Geometry: final body of the model. Coordinates: model frame, mm. A direction names the side the tool comes from. Round coordinates to 2 decimals unless told otherwise and drop trailing zeros. Loops run counter-clockwise (first coordinate to the right, second up) from the corner with the lowest first, then second, coordinate; pieces in that order, holes last. Notation, with made-up numbers: (-9, 79) - (22, 79) arc R21 cw to (22, 92) - close; hole circle Ø4 at (-40, -23.75). An arc over 180 degrees is marked (long way). Return JSON: item names as keys, results as strings. Group by question number.
1. Set-up query: faces 1 (the face through (-1, 0, 5)), 2 (the face through (14.53, 14.55, 2.54)), 3 (the face through (37, 27.5, 3)). Return all of +Z, -Z, +X, -X, +Y, -Y with unobstructed straight access to the full face (end or side cutting, diameter ignored); none if empty.
2. Material intervals for probe 1 along X at (y, z) = (12, 13); probe 2 along Y at (x, z) = (-1.5, 7); probe 3 along X at (y, z) = (18, 4.5), sorted ascending.
3. Section B-B on x = -50. Return loops of the section in (y, z), and give its area (3 significant figures).
4. Section D-D on x = 7.5. Return loops of the section in (y, z).
5. Section A-A on z = 18.5. Return loops of the section in (x, y), and give its area (3 significant figures).
6. Draft query along X for faces 4 (the face through (21.86, 9.83, 2.54)), 5 (the face through (-20, 29, 4)), 6 (the face through (0, 30.5, 4)). Return one class per face: +X half, -X half, draft (parallel to the pull), parting line (faces both ways), or undercut.
7. First-contact query: pin 1 Ø6 at (x, y) = (33.5, -0.5) entering from +Z; pin 2 Ø1.5 at (y, z) = (29, 2) entering from +X; pin 3 Ø3.5 at (y, z) = (29, 2.5) entering from -X. Flat tips, straight axial feed; report the tip coordinate or a pass-through.
from build123d import *

# Parameters (mm, degrees)
SKETCH1_W             = 82
SKETCH1_H             = 55
BOSS_EXTRUDE1_DEPTH   = 5
SKETCH1_W_2           = 12
BOSS_EXTRUDE1_2_DEPTH = 5
BOSS_EXTRUDE1_3_DEPTH = 5
SKETCH1_3_W           = 2
SKETCH1_3_H           = 55
BOSS_EXTRUDE2_DEPTH   = 7
FILLET1_R             = 1
SKETCH2_W             = 5
SKETCH2_H             = 45
BOSS_EXTRUDE3_DEPTH   = 16
SKETCH3_W             = 17
SKETCH3_H             = 45
BOSS_EXTRUDE4_DEPTH   = 5
SKETCH4_W             = 40
SKETCH4_H             = 3
BOSS_EXTRUDE5_DEPTH   = 8
CUT_EXTRUDE1_DEPTH    = 8


with BuildPart() as part:
    # Sketch1 → Boss-Extrude1 (new body)
    with BuildSketch(Plane.XY):
        Rectangle(SKETCH1_W, SKETCH1_H)
    extrude(amount=BOSS_EXTRUDE1_DEPTH)



with BuildPart() as body_2:
    # Sketch1 → Boss-Extrude1 2 (new body)
    with BuildSketch(Plane.XY):
        with Locations((-49, 0)):
            Rectangle(SKETCH1_W_2, SKETCH1_H)
    extrude(amount=BOSS_EXTRUDE1_2_DEPTH)


with BuildPart() as body_3:
    # Sketch1 → Boss-Extrude1 3 (new body)
    with BuildSketch(Plane.XY):
        with Locations((49, 0)):
            Rectangle(SKETCH1_W_2, SKETCH1_H)
    extrude(amount=BOSS_EXTRUDE1_3_DEPTH)


with BuildPart() as part_1:
    add(part.part)

    add(body_2.part)  # Boss-Extrude2 merges body 2

    add(body_3.part)  # Boss-Extrude2 merges body 3
    # Sketch1<3> → Boss-Extrude2 (add)
    with BuildSketch(Plane.XY):
        with Locations((42, 0)):
            Rectangle(SKETCH1_3_W, SKETCH1_3_H)
        with Locations((-42, 0)):
            Rectangle(SKETCH1_3_W, SKETCH1_3_H)
    extrude(amount=BOSS_EXTRUDE2_DEPTH)

    # Fillet1
    fillet1_edges = [part_1.edges().sort_by_distance(p)[0] for p in [
        (-43, 0, 7),
        (-41, 0, 7),
        (41, 0, 7),
        (43, 0, 7),
    ]]
    fillet(fillet1_edges, radius=FILLET1_R - 0.0001)  # a hair under: the kernel refuses the full size

    # Sketch2 → Boss-Extrude3 (add)
    with BuildSketch(Plane.XY):
        with Locations((-57.5, 0)):
            Rectangle(SKETCH2_W, SKETCH2_H)
        with Locations((57.5, 0)):
            Rectangle(SKETCH2_W, SKETCH2_H)
    extrude(amount=BOSS_EXTRUDE3_DEPTH)

    # Sketch3 → Boss-Extrude4 (add)
    with BuildSketch(Plane.XY.offset(16)):
        with Locations((51.5, 0)):
            Rectangle(SKETCH3_W, SKETCH3_H)
        with Locations((-51.5, 0)):
            Rectangle(SKETCH3_W, SKETCH3_H)
    extrude(amount=BOSS_EXTRUDE4_DEPTH)

    # Sketch4 → Boss-Extrude5 (add)
    with BuildSketch(Plane.XY):
        with Locations((0, -29)):
            Rectangle(SKETCH4_W, SKETCH4_H)
        with Locations((0, 29)):
            Rectangle(SKETCH4_W, SKETCH4_H)
    extrude(amount=BOSS_EXTRUDE5_DEPTH)

    # Sketch5 → Cut-Extrude1 (cut)
    with BuildSketch(Plane.XY.offset(5)):
        Polygon((32.5, -2.5), (11.171238341, -2.5), (32.5, -16.386089579), align=None)
        Polygon((26.151212641, -21.798780488), (4, -7.377234224), (4, -21.798780488), align=None)
        Polygon((-4, -7.494684737), (-25.350036879, -21.798780488), (-4, -21.798780488), align=None)
        Polygon((-10.917888224, -2.5), (-32.5, -2.5), (-32.5, -16.959581269), align=None)
        Polygon((-11.171238341, 2.5), (-32.5, 16.386089579), (-32.5, 2.5), align=None)
        Polygon((-4, 21.798780488), (-26.151212641, 21.798780488), (-4, 7.377234224), align=None)
        Polygon((25.350035913, 21.798780488), (4, 21.798780488), (4, 7.494685385), align=None)
        Polygon((32.5, 2.5), (32.5, 16.959581917), (10.917887257, 2.5), align=None)
    extrude(amount=-CUT_EXTRUDE1_DEPTH, mode=Mode.SUBTRACT)


solid = part_1.part
Taken from the geometry:
{
 "1": {"face 1": "+Z", "face 2": "+Z, -Z", "face 3": "+Z, -Z, +X, +Y"},
 "2": {"probe 1": "-60 to -55, 55 to 60", "probe 2": "-30.5 to -27.5, 27.5 to 30.5", "probe 3": "-60 to -20.32, -4 to 4, 19.68 to 60"},
 "3": {"outline": "(-27.5, 0) - (27.5, 0) - (27.5, 5) - (-27.5, 5) - close; (-22.5, 16) - (22.5, 16) - (22.5, 21) - (-22.5, 21) - close", "area": "500 mm2"},
 "4": {"outline": "(-30.5, 0) - (-21.8, 0) - (-21.8, 5) - (-27.5, 5) - (-27.5, 8) - (-30.5, 8) - close; (-9.66, 0) - (9.84, 0) - (9.84, 5) - (-9.66, 5) - close; (21.8, 0) - (30.5, 0) - (30.5, 8) - (27.5, 8) - (27.5, 5) - (21.8, 5) - close"},
 "5": {"outline": "(-60, -22.5) - (-43, -22.5) - (-43, 22.5) - (-60, 22.5) - close; (43, -22.5) - (60, -22.5) - (60, 22.5) - (43, 22.5) - close", "area": "1,530 mm2"},
 "6": {"face 4": "undercut", "face 5": "-X half", "face 6": "draft"},
 "7": {"pin 1": "z = 5", "pin 2": "x = 20", "pin 3": "x = -55"}
}
